Work out the finished part from the listing and answer in its coordinate system (mm). Give positions to 0.01 mm unless a question says otherwise; leave off trailing zeros. Order: outer loops, then holes, each group sorted by start corner. A loop starts at its lowest first (then second) coordinate and runs counter-clockwise, first axis right, second up.
```python
from build123d import *

# Parameters (mm, degrees)
ESBO_O1_W                = 300
ESBO_O1_H                = 180
ESBO_O1_R                = 1.5
ESBO_O1_R_2              = 2
ESBO_O1_R_3              = 15
ESBO_O1_R_4              = 4
ESBO_O1_R_5              = 1.65
ESBO_O1_W_2              = 20
ESBO_O1_H_2              = 20
RESSALTO_EXTRUS_O1_DEPTH = 6
ESBO_O2_R                = 2
CORTE_EXTRUS_O1_DEPTH    = 10
ESBO_O3_R                = 2
CORTE_EXTRUS_O2_DEPTH    = 10


with BuildPart() as part:
    # Esboço1 → Ressalto-extrusão1 (new body)
    with BuildSketch(Plane.XY):
        Rectangle(ESBO_O1_W, ESBO_O1_H)
        with Locations((140, 5)):
            Circle(ESBO_O1_R, mode=Mode.SUBTRACT)
        with Locations((140, -80)):
            Circle(ESBO_O1_R, mode=Mode.SUBTRACT)
        with Locations((60, -80)):
            Circle(ESBO_O1_R, mode=Mode.SUBTRACT)
        with Locations((60, 5)):
            Circle(ESBO_O1_R, mode=Mode.SUBTRACT)
        with Locations((-110, -56.5)):
            Circle(ESBO_O1_R_2, mode=Mode.SUBTRACT)
        with Locations((-40, -56.5)):
            Circle(ESBO_O1_R_2, mode=Mode.SUBTRACT)
        with Locations((-75, -64)):
            Circle(ESBO_O1_R_3, mode=Mode.SUBTRACT)
        with Locations((-35, -64)):
            Circle(ESBO_O1_R_4, mode=Mode.SUBTRACT)
        with Locations((-115, -64)):
            Circle(ESBO_O1_R_4, mode=Mode.SUBTRACT)
        with Locations((-40, -71.5)):
            Circle(ESBO_O1_R_2, mode=Mode.SUBTRACT)
        with Locations((-110, -71.5)):
            Circle(ESBO_O1_R_2, mode=Mode.SUBTRACT)
        with Locations((35, -3)):
            Circle(ESBO_O1_R_5, mode=Mode.SUBTRACT)
        with Locations((35, -28)):
            Circle(ESBO_O1_R_5, mode=Mode.SUBTRACT)
        with Locations((-130, 60)):
            Circle(ESBO_O1_R_5, mode=Mode.SUBTRACT)
        with Locations((-20, 60)):
            Circle(ESBO_O1_R_5, mode=Mode.SUBTRACT)
        with Locations((-20, 5)):
            Circle(ESBO_O1_R_5, mode=Mode.SUBTRACT)
        with Locations((-130, 5)):
            Circle(ESBO_O1_R_5, mode=Mode.SUBTRACT)
        with Locations((100, -51.75)):
            Rectangle(ESBO_O1_W_2, ESBO_O1_H_2, mode=Mode.SUBTRACT)
    extrude(amount=RESSALTO_EXTRUS_O1_DEPTH)

    # Esboço2 → Corte-extrusão1 (cut)
    with BuildSketch(Plane.XY.offset(6)):
        with Locations((-140, 80)):
            Circle(ESBO_O2_R)
        with Locations((140, 80)):
            Circle(ESBO_O2_R)
        with Locations((120, -80)):
            Circle(ESBO_O2_R)
        with Locations((-140, -80)):
            Circle(ESBO_O2_R)
    extrude(amount=-CORTE_EXTRUS_O1_DEPTH, mode=Mode.SUBTRACT)

    # Esboço3 → Corte-extrusão2 (cut)
    with BuildSketch(Plane.XY.offset(6)):
        with Locations((105, -67.5)):
            Circle(ESBO_O3_R)
        with Locations((105, -36.5)):
            Circle(ESBO_O3_R)
        with Locations((95, -36.5)):
            Circle(ESBO_O3_R)
        with Locations((95, -67.5)):
            Circle(ESBO_O3_R)
    extrude(amount=-CORTE_EXTRUS_O2_DEPTH, mode=Mode.SUBTRACT)


solid = part.part
```
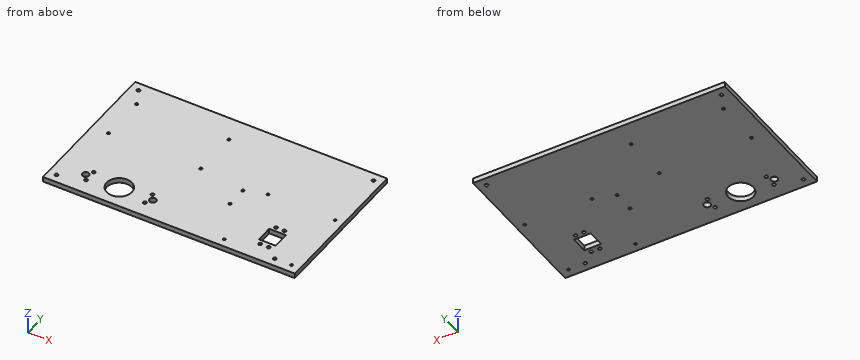
1. Straight lines are drawn through the part: probe 1 along Y at (x, z) = (-140, 3.9); probe 2 along Y at (x, z) = (-40, 2.2); probe 3 along Y at (x, z) = (119.5, 3.15). For each, find the intervals that lie inside material, in ascending order.
Findings below:
probe 1: y = -90 to -82, -78 to 78, 82 to 90
probe 2: y = -90 to -73.5, -69.5 to -58.5, -54.5 to 90
probe 3: y = -90 to -81.94, -78.06 to 90
2. Given P1, Ø3.5, axis at x = -40, y = -56.5, coming from the +Z side; P2, Ø4.5, axis at x = -20, y = 60, coming from the +Z side, each flat-ended and moving along its own axis, determine where each tip first touches the part or whether it passes through.
Findings below:
P1: passes through
P2: stops at z = 6
3. The part is cut by section A-A (z = 0.95). State how many separate pieces and enclosed holes the cut face has, then the cut area to 3 significant figures.
Findings below:
separate pieces: 1
enclosed holes: 26
area: 52,600 mm2
4. The part is cut by section B-B (x = -72). Write down the section's boundary in (y, z).
Findings below:
outline: (-90, 0) - (-78.7, 0) - (-78.7, 6) - (-90, 6) - close; (-49.3, 0) - (90, 0) - (90, 6) - (-49.3, 6) - close
